Check sheet for the modelled part. Datum: model origin and axes. Units: mm. Round coordinates to 2 decimals unless told otherwise and drop trailing zeros. Order: outer loops, then holes, each group sorted by start corner. A loop starts at its lowest first (then second) coordinate and runs counter-clockwise, first axis right, second up.
(1) Sectioned sample at D-D, the plane z = 2. Enter the section's corners in (x, y).
(2) Sectioned sample at A-A, the plane y = 0. Enter the section's corners in (x, z).
(3) Mould release check, pull along Y, two halves, no side actions. Record for faces 1 (the cylindrical face through (-6.944, -5.324, 4.938)), 2 (the flat face through (0, 0, 0)), 3 (the cylindrical face through (-7.493, 0.33, 5.902)): released by +Y, released by -Y, zero draft, split by the parting line, or undercut.
(4) Sectioned sample at B-B, the plane z = 4. Enter the section's corners in (x, y).
(5) Thickness scan on probe 1 along Y at (x, z) = (0, 6.25); probe 2 along Z at (x, y) = (-4, -1); probe 3 along X at (y, z) = (-5.75, 7.5). Record the ranges inside material, lowest first.
(6) Depth check by flat-ended pin: pin 1 (4 mm diameter, centred on y = 4.5, z = 5.5, fed in from +X); pin 2 (3 mm diameter, centred on x = 1, y = -2, fed in from +Z); pin 3 (1 mm diameter, centred on y = 6, z = 3, fed in from -X). Enter the tip coordinate at first touch or a pass-through.
```python
from build123d import *

# Parameters (mm, degrees)
F0_R     = 7.5
F1_DEPTH = 2.5
F0_R_2   = 8.75
F2_DEPTH = 10
F3_R     = 0.6


with BuildPart() as f1:
    # F0 (on Top) → F1 (new body)
    with BuildSketch(Plane.XY):
        Circle(F0_R)
    extrude(amount=F1_DEPTH)

    # F0 (on Top) → F2 (join)
    with BuildSketch(Plane.XY):
        Circle(F0_R_2)
        Circle(F0_R, mode=Mode.SUBTRACT)
    extrude(amount=F2_DEPTH)

    # F3
    f3_edges = [f1.edges().sort_by_distance(p)[0] for p in [
        (-7.5, 0, 10),
        (-8.75, 0, 10),
        (-8.75, 0, 0),
    ]]
    fillet(f3_edges, radius=F3_R)


solid = f1.part
```
Derived:
1. outline: circle Ø17.5 at (0, 0)
2. outline: (-8.75, 0.6) arc R0.6 ccw to (-8.15, 0) - (8.15, 0) arc R0.6 ccw to (8.75, 0.6) - (8.75, 9.4) arc R0.6 ccw to (8.15, 10) - (8.1, 10) arc R0.6 ccw to (7.5, 9.4) - (7.5, 2.5) - (-7.5, 2.5) - (-7.5, 9.4) arc R0.6 ccw to (-8.1, 10) - (-8.15, 10) arc R0.6 ccw to (-8.75, 9.4) - close
3. face 1: split by the parting line
3. face 2: zero draft
3. face 3: undercut
4. outline: circle Ø17.5 at (0, 0); hole circle Ø15 at (0, 0)
5. probe 1: y = -8.75 to -7.5, 7.5 to 8.75
5. probe 2: z = 0 to 2.5
5. probe 3: x = -6.6 to -4.82, 4.82 to 6.6
6. pin 1: stops at x = 8.39
6. pin 2: stops at z = 2.5
6. pin 3: stops at x = -6.81
